Can you work these out from the model? Positions are in its coordinate system, mm. A direction names the side the tool comes from. Round coordinates to 2 decimals unless told otherwise and drop trailing zeros. Loops run counter-clockwise (first coordinate to the right, second up) from the corner with the lowest first, then second, coordinate; pieces in that order, holes last.
Autodesk Inventor part; units mm, degrees
ref_plane "YZ Plane" through (0, 0, 0) normal (1, 0, 0) x (0, 1, 0)
ref_plane "XZ Plane" through (0, 0, 0) normal (0, 1, 0) x (-1, 0, 0)
ref_plane "XY Plane" through (0, 0, 0) normal (0, 0, 1) x (1, 0, 0)
sketch "Sketch1" plane through (0, 0, 0) normal (0, 1, 0) x (-1, 0, 0)
  line L0 (16.375, 22.625) -> (-16.375, 22.625)
  line L1 (-16.375, 22.625) -> (-16.375, -22.625)
  line L2 (-16.375, -22.625) -> (16.375, -22.625)
  line L3 (16.375, -22.625) -> (16.375, 22.625)
  line L4 (16.375, 22.625) -> (-16.375, -22.625) construction
  line L5 (-16.375, 22.625) -> (16.375, -22.625) construction
  point P0 (0, 0)
  dimension "d0" = 32.75
  dimension "d1" = 45.25
extrude "Extrusion1" add sketch "Sketch1" along normal blind 12
sketch "Sketch2" plane through (0, 12, 0) normal (0, 1, 0) x (1, 0, 0)
  line L0 (-15.375, -21.625) -> (15.375, -21.625)
  line L1 (15.375, -21.625) -> (15.375, 21.625)
  line L2 (15.375, 21.625) -> (-15.375, 21.625)
  line L3 (-15.375, 21.625) -> (-15.375, -21.625)
  line L4 (-15.375, -21.625) -> (15.375, 21.625) construction
  line L5 (15.375, -21.625) -> (-15.375, 21.625) construction
  point P0 (0, 0)
  dimension "d4" = 30.75
  dimension "d5" = 43.25
extrude "Extrusion2" cut sketch "Sketch2" against normal blind 11
sketch "Sketch5" plane through (0, 1, 0) normal (0, 1, 0) x (1, 0, 0)
  circle A0 centre (12.625, 18.875) radius 2
  circle A1 centre (-12.625, -18.875) radius 2
  line L0 (15.375, 21.625) -> (15.375, -21.625)
  line L1 (-15.375, 21.625) -> (15.375, 21.625)
  line L2 (-15.375, -21.625) -> (-15.375, 21.625)
  line L3 (15.375, -21.625) -> (-15.375, -21.625)
  point P0 (0, 0)
  dimension "d20" = 4
  dimension "d21" = 2.75
  dimension "d22" = 2.75
  dimension "d23" = 2.75
  dimension "d24" = 2.75
  dimension "d25" = 4
extrude "Extrusion5" add sketch "Sketch5" along normal blind 10 contours A0 | A1
sketch "Sketch6" plane through (12.625, 11, -18.875) normal (0, 1, 0) x (1, 0, 0)
  circle A0 centre (-25.25, -37.75) radius 2
  circle A1 centre (-25.25, -37.75) radius 1
  circle A2 centre (0, 0) radius 2
  circle A3 centre (0, 0) radius 1
  point P0 (-12.625, -18.875)
  dimension "d28" = 2
  dimension "d29" = 2
extrude "Extrusion6" cut sketch "Sketch6" against normal blind 10 contours A1 | A3
sketch "Sketch7" plane through (0, 12, 0) normal (0, 1, 0) x (1, 0, 0)
  line L0 (16.375, 22.625) -> (-16.375, 22.625)
  line L1 (-15.375, 21.625) -> (-2.875, 21.625)
  line L2 (-2.875, 21.625) -> (-2.875, 22.625)
  line L3 (-2.875, 22.625) -> (-15.375, 22.625)
  line L4 (-15.375, 22.625) -> (-15.375, 21.625)
  line L5 (15.375, -21.625) -> (-15.375, -21.625)
  line L6 (-16.375, -22.625) -> (16.375, -22.625)
  line L7 (-9.875, -21.625) -> (6.625, -21.625)
  line L8 (6.625, -21.625) -> (6.625, -22.625)
  line L9 (6.625, -22.625) -> (-9.875, -22.625)
  line L10 (-9.875, -22.625) -> (-9.875, -21.625)
  line L11 (-15.375, -21.625) -> (-15.375, 21.625)
  point P0 (0, 0)
  dimension "d32" = 12.5
  dimension "d33" = 5.5
  dimension "d35" = 22
extrude "Extrusion7" cut sketch "Sketch7" against normal blind 11
sketch "Sketch8" plane through (0, 0, 0) normal (0, -1, 0) x (1, 0, 0)
  line L0 (16.375, 22.625) -> (16.375, -22.625)
  line L1 (16.375, 7.5) -> (31.375, 7.5)
  line L2 (31.375, 7.5) -> (31.375, -7.5)
  line L3 (31.375, -7.5) -> (16.375, -7.5)
  line L4 (16.375, -7.5) -> (16.375, 7.5)
  point P0 (0, 0)
  dimension "d38" = 15
  dimension "d39" = 7.5
  dimension "d40" = 15
extrude "Extrusion8" add sketch "Sketch8" against normal blind 8
sketch "Sketch9" plane through (0, 8, 0) normal (0, 1, 0) x (1, 0, 0)
  line L0 (31.375, -7.5) -> (31.375, 7.5)
  point P0 (0, 0)
  point P1 (23.875, 0.0223)
  dimension "d50" = 7.5
hole "Hole1" at (23.875, 8, -0.0223) direction (0, -1, 0) diameter 6.756 depth 10.9728 tip angle 118 counterbore diameter 11.113 counterbore depth 6.35
fillet "Fillet1" radius 3 2 edges at (16.375, 4, -7.5) (16.375, 4, 7.5)
fillet "Fillet2" radius 7.5 2 edges at (31.375, 4, -7.5) (31.375, 4, 7.5)
properties part number "ResonanceBoardEnc"
(1) For faces 4 (the cylindrical face through (21.027, 0.813, 1.794)), 5 (the flat face through (-15.375, 7, -1)), 6 (the flat face through (13, 1, -19)), 7 (the flat face through (18, 8, -1)), 8 (the flat face through (16.375, 9, 0)), which set-ups out of +Z, -Z, +X, -X, +Y, -Y let a thin tool reach every point of the face, with its end or its side?
Worked answers:
face 4: +Y, -Y
face 5: -Z, +Y
face 6: +Y
face 7: +Z, -Z, +X, +Y
face 8: +X, +Y
(2) If we section it at B-B, the plane x = 7.5: List the corners of the cut face in (y, z) for me (3 decimals).
Worked answers:
outline: (0, -22.625) - (12, -22.625) - (12, -21.625) - (1, -21.625) - (1, 21.625) - (12, 21.625) - (12, 22.625) - (0, 22.625) - close
(3) If we section it at C-C, the plane z = -1: List the corners of the cut face in (x, y) for me (3 decimals), then the cut area to 3 significant figures.
Worked answers:
outline: (-16.375, 0) - (20.642, 0) - (20.642, 1.65) - (18.405, 1.65) - (18.405, 8) - (16.375, 8) - (16.375, 12) - (15.375, 12) - (15.375, 1) - (-15.375, 1) - (-15.375, 12) - (-16.375, 12) - close; (27.108, 0) - (31.308, 0) - (31.308, 8) - (29.345, 8) - (29.345, 1.65) - (27.108, 1.65) - close
area: 94.1 mm2
(4) If I drill on line 1 (X direction, y = 2.5, z = -19) (3 decimals); line 2 (Z direction, x = 24, y = 6.25); line 3 (X direction, y = 11.25, z = -15) (3 decimals), over which ranges is the centre line in solid material (lowest first)?
Worked answers:
line 1: x = -16.375 to -15.375, 10.629 to 11.633, 13.617 to 14.621, 15.375 to 16.375
line 2: z = -7.5 to -5.58, 5.53 to 7.5
line 3: x = -16.375 to -15.375, 15.375 to 16.375
(5) If we section it at A-A, the plane y = 9: List the corners of the cut face in (x, z) for me (3 decimals).
Worked answers:
outline: (-16.375, -22.625) - (-15.375, -22.625) - (-15.375, 21.625) - (-9.875, 21.625) - (-9.875, 22.625) - (-16.375, 22.625) - close; circle Ø4 at (-12.625, 18.875); (-2.875, -22.625) - (16.375, -22.625) - (16.375, 22.625) - (6.625, 22.625) - (6.625, 21.625) - (15.375, 21.625) - (15.375, -21.625) - (-2.875, -21.625) - close; circle Ø4 at (12.625, -18.875); hole circle Ø2 at (-12.625, 18.875); hole circle Ø2 at (12.625, -18.875)
(6) If we mould it in two halves opening along X, with no side actions, what happens to faces 1 (the cylindrical face through (29.24, 4.06, -5.24)), 2 (the flat face through (6, 7, -21.625)), 3 (the flat face through (8, 6, -22.625))? For each: released by +X, released by -X, zero draft, split by the parting line, or undercut.
Worked answers:
face 1: released by +X
face 2: undercut
face 3: zero draft
(7) Will these pins go through, and if not, where does the flat tip stop? P1, Ø1.8, axis at x = 12.625, z = -18.875, coming from the +Y side; P2, Ø5.5, axis at y = 8, z = -4.5, coming from the +X side; P3, Ø12, axis at x = 22.5, z = -2, coming from the +Y side.
Worked answers:
P1: stops at y = 1
P2: stops at x = 31.17
P3: stops at y = 8
(8) If we section it at D-D, the plane x = 25: List the corners of the cut face in (y, z) for me.
Worked answers:
outline: (0, -7.42) - (8, -7.42) - (8, -5.46) - (1.65, -5.46) - (1.65, -3.21) - (0, -3.21) - close; (0, 3.16) - (1.65, 3.16) - (1.65, 5.42) - (8, 5.42) - (8, 7.42) - (0, 7.42) - close
